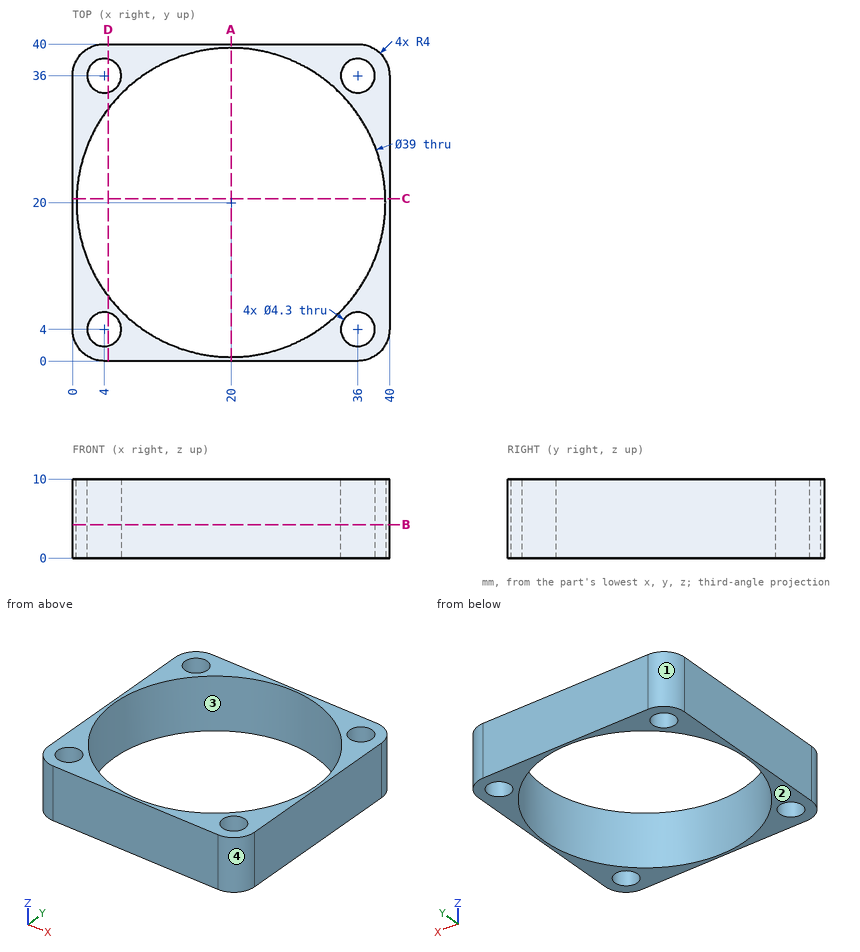
Drawing for the job (mm, zero at the part's lowest x, y, z). Coordinates: 2 decimals unless noted, no trailing zeros. Write each loop counter-clockwise with the first axis right and the second up, starting at its lowest first coordinate (ties: lowest second). Pieces come first, ordered by that corner, then holes. Notation, with made-up numbers: (23, 44) -> (66, 44) arc R20 cw to (66, 83) -> close; hole circle Ø3 at (3.5, -34.5). An arc over 180 degrees is marked (long way). One line per item, written item: value. Start each with the question number.
1) Slice it at D-D on x = 4.5. Write the cut outline in (y, z), then the cut area to 3 significant figures.
2) Probe probe 1 along Y at (x, z) = (20, 6.5); probe 2 along X at (y, z) = (19.5, 3); probe 3 along Y at (x, z) = (37, 6.75). List the from-to ranges inside material, lowest first.
3) Slice it at A-A on x = 20. Write the cut outline in (y, z), then the cut area to 3 significant figures.
4) Slice it at B-B on z = 4.25. Write the cut outline in (x, y).
5) Flat gauge pin, fed straight in: pin 1 Ø12 at (x, y) = (26, 27.5) entering from -Z. Where does the tip first touch, or does it go through?
6) Pull direction X, two halves, no side cores. Call the marked faces 1, 2, 3 and 4: +X half, -X half, draft (parallel to the pull), parting line (faces both ways), or undercut.
7) Slice it at C-C on y = 20.5. Write the cut outline in (x, z), then the cut area to 3 significant figures.
Answers follow:
1. outline: (0, 0) -> (1.91, 0) -> (1.91, 10) -> (0, 10) -> close; (6.09, 0) -> (8.17, 0) -> (8.17, 10) -> (6.09, 10) -> close; (31.83, 0) -> (33.91, 0) -> (33.91, 10) -> (31.83, 10) -> close; (38.09, 0) -> (40, 0) -> (40, 10) -> (38.09, 10) -> close
1. area: 79.7 mm2
2. probe 1: 0 to 0.5, 39.5 to 40
2. probe 2: 0 to 0.51, 39.49 to 40
2. probe 3: 0.13 to 2.1, 5.9 to 10.45, 29.55 to 34.1, 37.9 to 39.87
3. outline: (0, 0) -> (0.5, 0) -> (0.5, 10) -> (0, 10) -> close; (39.5, 0) -> (40, 0) -> (40, 10) -> (39.5, 10) -> close
3. area: 10.0 mm2
4. outline: (0, 4) arc R4 ccw to (4, 0) -> (36, 0) arc R4 ccw to (40, 4) -> (40, 36) arc R4 ccw to (36, 40) -> (4, 40) arc R4 ccw to (0, 36) -> close; hole circle Ø39 at (20, 20); hole circle Ø4.3 at (4, 4); hole circle Ø4.3 at (4, 36); hole circle Ø4.3 at (36, 4); hole circle Ø4.3 at (36, 36)
5. pin 1: through
6. face 1: -X half
6. face 2: draft
6. face 3: undercut
6. face 4: +X half
7. outline: (0, 0) -> (0.51, 0) -> (0.51, 10) -> (0, 10) -> close; (39.49, 0) -> (40, 0) -> (40, 10) -> (39.49, 10) -> close
7. area: 10.1 mm2
